```python
from build123d import *

# Parameters (mm, degrees)
ESQUISSE1_R             = 25
BOSS_EXTRU_1_DEPTH      = 2
ENL_V_MAT_EXTRU_1_REACH = 37.412
ESQUISSE2_W             = 11.684
ESQUISSE2_H             = 23.749


with BuildPart() as part:
    # Esquisse1 → Boss.-Extru.1 (new body)
    with BuildSketch(Plane.XY):
        Circle(ESQUISSE1_R)
    extrude(amount=BOSS_EXTRU_1_DEPTH)

    # Esquisse2 → Enlèv. mat.-Extru.1 (cut, up to next)
    with BuildSketch(Plane.XY.offset(2), mode=Mode.PRIVATE) as enl_v_mat_extru_1_sk1:
        Rectangle(ESQUISSE2_W, ESQUISSE2_H)
    enl_v_mat_extru_1_tool1 = extrude(enl_v_mat_extru_1_sk1.sketch, amount=-ENL_V_MAT_EXTRU_1_REACH, mode=Mode.PRIVATE) & part.part
    add(enl_v_mat_extru_1_tool1.solids().sort_by_distance((0, 0, 2))[0], mode=Mode.SUBTRACT)


solid = part.part
```
Verification items for the finished model (mm, model axes). A direction names the side the tool comes from. Coordinates: 2 decimals unless noted, no trailing zeros. Loops run counter-clockwise (first coordinate to the right, second up) from the corner with the lowest first, then second, coordinate; pieces in that order, holes last. Notation, with made-up numbers: (61.5, 65) -> (81.5, 65) arc R9 ccw to (81.5, 77) -> close; hole circle Ø6 at (42.5, 60). An arc over 180 degrees is marked (long way). Answer in a Markdown table with one row per item. Add a question column.
1. Depth check by flat-ended pin: P1, Ø1, axis at x = 5.5, y = -10, coming from the +Z side; P2, Ø1, axis at x = 3, z = 0.5, coming from the -Y side; P3, Ø0.6, axis at y = 2, z = 1, coming from the +X side; P4, Ø1, axis at x = 1, z = 1, coming from the -Y side (3 decimals). Enter the tip coordinate at first touch or a pass-through.
2. Section check A-A, the plane x = 0. Enter the section's corners in (y, z), then the cut area to 3 significant figures.
3. Section check C-C, the plane z = 0.95. Enter the section's corners in (x, y).
4. Access from +Z, -Z, +X, -X, +Y, -Y to the whole of each face (thin tool, end or side, straight path). Record for faces 1 (the face through (-6, 0, 2)), 2 (the face through (5.842, 0, 1)).
5. Section check B-B, the plane y = 0. Enter the section's corners in (x, z), then the cut area to 3 significant figures.
6. Section check D-D, the plane y = 15. Enter the section's corners in (x, z).
7. Material ranges on probe 1 along Y at (x, z) = (0.5, 1.75) (1 decimal); probe 2 along X at (y, z) = (1, 1.4); probe 3 along X at (y, z) = (9.5, 1.3), recorded low to high. Write a range as [from, to].
8. Draft check along Y on faces 3 (the face through (-6, 0, 0)), 4 (the face through (23.846, 7.509, 0.986)), 5 (the face through (0, 11.874, 1)). Enter one of: +Y half, -Y half, draft (parallel to the pull), parting line (faces both ways), or undercut.
Derived:
| question | item | result |
|---|---|---|
| 1 | P1 | stops at z = 2 |
| 1 | P2 | stops at y = -24.87 |
| 1 | P3 | stops at x = 24.94 |
| 1 | P4 | stops at y = -24.995 |
| 2 | outline | (-25, 0) -> (-11.87, 0) -> (-11.87, 2) -> (-25, 2) -> close; (11.87, 0) -> (25, 0) -> (25, 2) -> (11.87, 2) -> close |
| 2 | area | 52.5 mm² |
| 3 | outline | circle Ø50 at (0, 0); hole (-5.84, -11.87) -> (5.84, -11.87) -> (5.84, 11.87) -> (-5.84, 11.87) -> close |
| 4 | face 1 | +Z, +X, -X, +Y, -Y |
| 4 | face 2 | +Z, -Z |
| 5 | outline | (-25, 0) -> (-5.84, 0) -> (-5.84, 2) -> (-25, 2) -> close; (5.84, 0) -> (25, 0) -> (25, 2) -> (5.84, 2) -> close |
| 5 | area | 76.6 mm² |
| 6 | outline | (-20, 0) -> (20, 0) -> (20, 2) -> (-20, 2) -> close |
| 7 | probe 1 | y = [-25, -11.9], [11.9, 25] |
| 7 | probe 2 | x = [-24.98, -5.84], [5.84, 24.98] |
| 7 | probe 3 | x = [-23.12, -5.84], [5.84, 23.12] |
| 8 | face 3 | draft |
| 8 | face 4 | parting line |
| 8 | face 5 | undercut |
